```python
from build123d import *

# Parameters (mm, degrees)
SKETCH1_W           = 105
SKETCH1_H           = 150
SKETCH1_W_2         = 5
SKETCH1_H_2         = 5
BOSS_EXTRUDE1_DEPTH = 35
SKETCH2_W           = 5
SKETCH2_H           = 5
SKETCH2_W_2         = 105
SKETCH2_H_2         = 150
BOSS_EXTRUDE2_DEPTH = 17.5
SKETCH3_W           = 105
SKETCH3_H           = 150
CUT_EXTRUDE1_DEPTH  = 47.5
CUT_EXTRUDE2_REACH  = 176.762
SKETCH4_R           = 6.5
CHAMFER1_SIZE       = 5
CHAMFER2_SIZE       = 5


with BuildPart() as part:
    # Sketch1 → Boss-Extrude1 (new body)
    with BuildSketch(Plane(origin=(0, 0, 0), x_dir=(1, 0, 0), z_dir=(0, 1, 0))):
        Polygon((52.5, -114.8421646), (-52.5, -114.8421646), (-52.5, 35.1578354), (-57.5, 35.1578354), (-57.5, -119.8421646), (52.5, -119.8421646), align=None)
        with Locations((0, -39.8421646)):
            Rectangle(SKETCH1_W, SKETCH1_H)
        Polygon((52.5, 35.1578354), (52.5, -114.8421646), (57.5, -114.8421646), (57.5, 40.1578354), (-52.5, 40.1578354), (-52.5, 35.1578354), align=None)
        with Locations((55, -117.3421646)):
            Rectangle(SKETCH1_W_2, SKETCH1_H_2)
        with Locations((-55, 37.6578354)):
            Rectangle(SKETCH1_W_2, SKETCH1_H_2)
    extrude(amount=BOSS_EXTRUDE1_DEPTH)

    # Sketch2 → Boss-Extrude2 (add)
    with BuildSketch(Plane(origin=(0, 35, 0), x_dir=(1, 0, 0), z_dir=(0, 1, 0))):
        Polygon((-77.5, -139.8421646), (-77.5, 35.1578354), (-77.5, 60.1578354), (-82.5, 60.1578354), (-82.5, -144.8421646), (77.5, -144.8421646), (77.5, -139.8421646), (52.5, -139.8421646), align=None)
        Polygon((-77.5, 60.1578354), (-52.5, 60.1578354), (77.5, 60.1578354), (77.5, -114.8421646), (77.5, -139.8421646), (82.5, -139.8421646), (82.5, 65.1578354), (-77.5, 65.1578354), align=None)
        with Locations((-80, 62.6578354)):
            Rectangle(SKETCH2_W, SKETCH2_H)
        Polygon((-77.5, 35.1578354), (-57.5, 35.1578354), (-57.5, 40.1578354), (-52.5, 40.1578354), (-52.5, 60.1578354), (-77.5, 60.1578354), align=None)
        Polygon((-52.5, 60.1578354), (-52.5, 40.1578354), (57.5, 40.1578354), (57.5, -114.8421646), (77.5, -114.8421646), (77.5, 60.1578354), align=None)
        Polygon((-52.5, 40.1578354), (-52.5, 35.1578354), (52.5, 35.1578354), (52.5, -114.8421646), (57.5, -114.8421646), (57.5, 40.1578354), align=None)
        with Locations((-55, 37.6578354)):
            Rectangle(SKETCH2_W, SKETCH2_H)
        Polygon((-52.5, -114.8421646), (-52.5, 35.1578354), (-57.5, 35.1578354), (-57.5, -119.8421646), (52.5, -119.8421646), (52.5, -114.8421646), align=None)
        Polygon((-57.5, -119.8421646), (-57.5, 35.1578354), (-77.5, 35.1578354), (-77.5, -139.8421646), (52.5, -139.8421646), (52.5, -119.8421646), align=None)
        with Locations((0, -39.8421646)):
            Rectangle(SKETCH2_W_2, SKETCH2_H_2)
        with Locations((55, -117.3421646)):
            Rectangle(SKETCH2_W, SKETCH2_H)
        Polygon((77.5, -114.8421646), (57.5, -114.8421646), (57.5, -119.8421646), (52.5, -119.8421646), (52.5, -139.8421646), (77.5, -139.8421646), align=None)
        with Locations((80, -142.3421646)):
            Rectangle(SKETCH2_W, SKETCH2_H)
    extrude(amount=BOSS_EXTRUDE2_DEPTH)

    # Sketch3 → Cut-Extrude1 (cut)
    with BuildSketch(Plane(origin=(0, 52.5, 0), x_dir=(1, 0, 0), z_dir=(0, 1, 0))):
        with Locations((0, -39.8421646)):
            Rectangle(SKETCH3_W, SKETCH3_H)
    extrude(amount=-CUT_EXTRUDE1_DEPTH, mode=Mode.SUBTRACT)

    # Sketch4 → Cut-Extrude2 (cut, up to next)
    with BuildSketch(Plane(origin=(0, 52.5, 0), x_dir=(1, 0, 0), z_dir=(0, 1, 0)), mode=Mode.PRIVATE) as cut_extrude2_sk1:
        with Locations(Location((-70, 52.6578354, 0), (0, 0, 270))):
            Circle(SKETCH4_R)
    cut_extrude2_tool1 = extrude(cut_extrude2_sk1.sketch, amount=-CUT_EXTRUDE2_REACH, mode=Mode.PRIVATE) & part.part
    # Sketch4 → Cut-Extrude2 (cut, up to next)
    with BuildSketch(Plane(origin=(0, 52.5, 0), x_dir=(1, 0, 0), z_dir=(0, 1, 0)), mode=Mode.PRIVATE) as cut_extrude2_sk2:
        with Locations(Location((-70, -132.3421646, 0), (0, 0, 270))):
            Circle(SKETCH4_R)
    cut_extrude2_tool2 = extrude(cut_extrude2_sk2.sketch, amount=-CUT_EXTRUDE2_REACH, mode=Mode.PRIVATE) & part.part
    # Sketch4 → Cut-Extrude2 (cut, up to next)
    with BuildSketch(Plane(origin=(0, 52.5, 0), x_dir=(1, 0, 0), z_dir=(0, 1, 0)), mode=Mode.PRIVATE) as cut_extrude2_sk3:
        with Locations(Location((70, -132.3421646, 0), (0, 0, 270))):
            Circle(SKETCH4_R)
    cut_extrude2_tool3 = extrude(cut_extrude2_sk3.sketch, amount=-CUT_EXTRUDE2_REACH, mode=Mode.PRIVATE) & part.part
    # Sketch4 → Cut-Extrude2 (cut, up to next)
    with BuildSketch(Plane(origin=(0, 52.5, 0), x_dir=(1, 0, 0), z_dir=(0, 1, 0)), mode=Mode.PRIVATE) as cut_extrude2_sk4:
        with Locations(Location((70, 52.6578354, 0), (0, 0, 270))):
            Circle(SKETCH4_R)
    cut_extrude2_tool4 = extrude(cut_extrude2_sk4.sketch, amount=-CUT_EXTRUDE2_REACH, mode=Mode.PRIVATE) & part.part
    add(cut_extrude2_tool1.solids().sort_by_distance((-70, 52.5, -52.657835))[0], mode=Mode.SUBTRACT)
    add(cut_extrude2_tool2.solids().sort_by_distance((-70, 52.5, 132.342165))[0], mode=Mode.SUBTRACT)
    add(cut_extrude2_tool3.solids().sort_by_distance((70, 52.5, 132.342165))[0], mode=Mode.SUBTRACT)
    add(cut_extrude2_tool4.solids().sort_by_distance((70, 52.5, -52.657835))[0], mode=Mode.SUBTRACT)

    # Chamfer1
    chamfer1_edges = [part.edges().sort_by_distance(p)[0] for p in [
        (0, 35, -40.1578354),
        (-57.5, 35, 39.8421646),
        (0, 35, 119.8421646),
        (57.5, 35, 39.8421646),
    ]]
    chamfer(chamfer1_edges, length=CHAMFER1_SIZE)

    # Chamfer2
    chamfer2_edges = [part.edges().sort_by_distance(p)[0] for p in [
        (82.5, 43.75, 144.8421646),
        (82.5, 43.75, -65.1578354),
        (-82.5, 43.75, -65.1578354),
        (-82.5, 43.75, 144.8421646),
    ]]
    chamfer(chamfer2_edges, length=CHAMFER2_SIZE)


solid = part.part
```
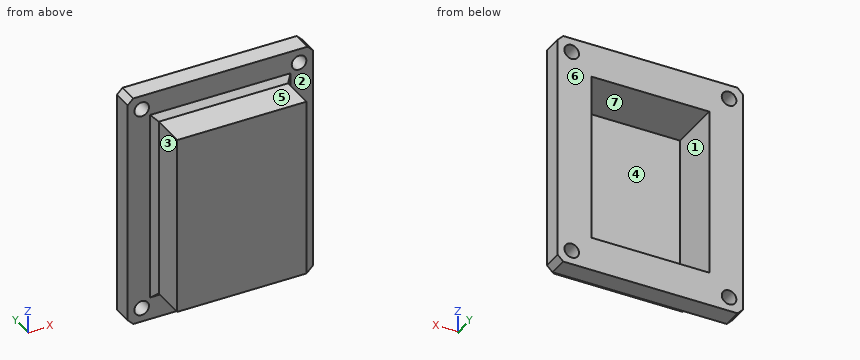
Part model, mm, in its own coordinate system. Face numbers are marked on the shaded views. A direction names the side the tool comes from. Round coordinates to 2 decimals unless told otherwise and drop trailing zeros. Loops run counter-clockwise (first coordinate to the right, second up) from the corner with the lowest first, then second, coordinate; pieces in that order, holes last. Notation, with made-up numbers: (45, -33.75) -> (69, -33.75) arc R25 ccw to (69, -2.75) -> close; hole circle Ø2 at (-38.5, 83). An arc over 180 degrees is marked (long way). Use one line per item in the form item = value. Start each with the question number.
Item 1: Drop flat-ended pins along their axis: pin 1 Ø1 at (y, z) = (20, 117) entering from +X; pin 2 Ø11.5 at (x, z) = (-70, -52.66) entering from +Y; pin 3 Ø2 at (x, z) = (19.5, 121) entering from -Y; pin 4 Ø3 at (x, y) = (-52, 5.5) entering from -Z. Give the stop position or say it passes through.
Item 2: Band-saw the part on A-A (x = -70). List the corners of the cut face in (y, z), plus the area to 3 significant figures.
Item 3: Band-saw the part on C-C (z = -24). List the corners of the cut face in (x, y).
Item 4: Band-saw the part on D-D (y = 41). List the corners of the cut face in (x, z), plus the area to 3 significant figures.
Item 5: Band-saw the part on B-B (y = 21.5). List the corners of the cut face in (x, z).
Item 6: Two-plate mould, pull along X, no slides. Class the marked faces 1, 2, 3 and 4: released by +X, released by -X, zero draft, split by the parting line, or undercut.
Item 7: Tool access for the marked faces 5, 6 and 7: list every direction of +Z, -Z, +X, -X, +Y, -Y with a clear straight run to the whole face (end or side of a thin tool).
Item 8: Drill centre lines: line 1 along X through (y, z) = (50, 132.5); line 2 along Z through (x, y) = (-30, 26.5); line 3 along X through (y, z) = (14, 48.5). Where is each one in solid material? Low to high.
Data:
q1.pin_1 = 57.5
q1.pin_2 = through
q1.pin_3 = 30.16
q1.pin_4 = -40.16
q2.outline = (35, -65.16) -> (52.5, -65.16) -> (52.5, -59.16) -> (35, -59.16) -> close; (35, -46.16) -> (52.5, -46.16) -> (52.5, 125.84) -> (35, 125.84) -> close; (35, 138.84) -> (52.5, 138.84) -> (52.5, 144.84) -> (35, 144.84) -> close
q2.area = 3,220 mm^2
q3.outline = (-82.5, 35) -> (-62.5, 35) -> (-57.5, 30) -> (-57.5, 0) -> (57.5, 0) -> (57.5, 30) -> (62.5, 35) -> (82.5, 35) -> (82.5, 52.5) -> (52.5, 52.5) -> (52.5, 5) -> (-52.5, 5) -> (-52.5, 52.5) -> (-82.5, 52.5) -> close
q4.outline = (-82.5, -60.16) -> (-77.5, -65.16) -> (77.5, -65.16) -> (82.5, -60.16) -> (82.5, 139.84) -> (77.5, 144.84) -> (-77.5, 144.84) -> (-82.5, 139.84) -> close; hole circle Ø13 at (-70, -52.66); hole circle Ø13 at (-70, 132.34); hole (-52.5, -35.16) -> (52.5, -35.16) -> (52.5, 114.84) -> (-52.5, 114.84) -> close; hole circle Ø13 at (70, -52.66); hole circle Ø13 at (70, 132.34)
q4.area = 18,300 mm^2
q5.outline = (-57.5, -40.16) -> (57.5, -40.16) -> (57.5, 119.84) -> (-57.5, 119.84) -> close; hole (-52.5, -35.16) -> (52.5, -35.16) -> (52.5, 114.84) -> (-52.5, 114.84) -> close
q6.face_1 = undercut
q6.face_2 = zero draft
q6.face_3 = released by -X
q6.face_4 = undercut
q7.face_5 = +Z, +X, -X, -Y
q7.face_6 = +Z, -Z, +X, -X, +Y
q7.face_7 = +Y
q8.line_1 = -82.5 to -76.5, -63.5 to 63.5, 76.5 to 82.5
q8.line_2 = -40.16 to -35.16, 114.84 to 119.84
q8.line_3 = -57.5 to -52.5, 52.5 to 57.5
